Source: CAD feature listing. Evaluate the final solid. Frame: model axes, mm. Coordinates: 2 decimals unless noted, no trailing zeros. Order: outer loops, then holes, each group sorted by start corner. A loop starts at its lowest first (then second) coordinate and runs counter-clockwise, first axis right, second up.
Item 1: Contact query for flat-ended pins moving along their axis: P1, Ø1.5, axis at x = -11, y = 2.5, coming from the -Z side (3 decimals); P2, Ø8, axis at x = -50, z = -52.5, coming from the -Y side; P3, Ø1, axis at y = 1, z = -73, coming from the +X side (3 decimals); P4, Ø1.6, axis at x = 1.5, y = 1, coming from the +Z side (3 decimals). Output: stop coordinate, or through.
Item 2: Section A-A on x = 0. Return the cut outline in (y, z) (3 decimals), then the cut area to 3 significant figures.
Item 3: Mould query, pull axis X, two halves, no side actions, for faces 1 (the flat face through (-68, 0, -46)), 2 (the cylindrical face through (-17.34, 1.61, 78.1)). Classes: released by +X, released by -X, zero draft, split by the parting line, or undercut.
Item 4: Section B-B on z = 0. Return the cut outline in (x, y) (3 decimals), then the cut area to 3 significant figures.
Item 5: Ray query, line 1 (Z direction, x = 0, y = 2.3) (3 decimals); line 2 (Z direction, x = -49.5, y = 3.05). Return the intervals inside material, ascending.
from build123d import *

# Parameters (mm, degrees)
ESQUISSE1_W             = 200
ESQUISSE1_H             = 200
BOSS_EXTRU_1_DEPTH      = 3.175
ESQUISSE2_W             = 3.175
ESQUISSE2_H             = 35
ESQUISSE2_H_2           = 47.5
ENL_V_MAT_EXTRU_1_DEPTH = 3.175
ESQUISSE4_W             = 44.325
ESQUISSE4_H             = 3.175
ESQUISSE4_W_2           = 35
ENL_V_MAT_EXTRU_3_DEPTH = 3.175
ESQUISSE3_R             = 80
ENL_V_MAT_EXTRU_2_DEPTH = 3.175


with BuildPart() as part:
    # Esquisse1 → Boss.-Extru.1 (new body)
    with BuildSketch(Plane(origin=(0, 0, 0), x_dir=(1, 0, 0), z_dir=(0, 1, 0))):
        Rectangle(ESQUISSE1_W, ESQUISSE1_H)
    extrude(amount=BOSS_EXTRU_1_DEPTH)

    # Esquisse2 → Enlèv. mat.-Extru.1 (cut)
    with BuildSketch(Plane(origin=(0, 3.175, 0), x_dir=(1, 0, 0), z_dir=(0, 1, 0))):
        with Locations((-98.4125, 0)):
            Rectangle(ESQUISSE2_W, ESQUISSE2_H)
        with Locations((-98.4125, 76.25)):
            Rectangle(ESQUISSE2_W, ESQUISSE2_H_2)
        with Locations((-98.4125, -76.25)):
            Rectangle(ESQUISSE2_W, ESQUISSE2_H_2)
    enl_v_mat_extru_1 = extrude(amount=-ENL_V_MAT_EXTRU_1_DEPTH, mode=Mode.SUBTRACT)

    # Symétrie1: Enlèv. mat.-Extru.1 across plane
    add(enl_v_mat_extru_1.mirror(Plane(origin=(0, 0, 0), x_dir=(0, 0, 1), z_dir=(1, 0, 0))), mode=Mode.SUBTRACT)

    # Esquisse4 → Enlèv. mat.-Extru.3 (cut)
    with BuildSketch(Plane(origin=(0, 3.175, 0), x_dir=(1, 0, 0), z_dir=(0, 1, 0))):
        with Locations((-74.6625, 98.4125)):
            Rectangle(ESQUISSE4_W, ESQUISSE4_H)
        with Locations((0, 98.4125)):
            Rectangle(ESQUISSE4_W_2, ESQUISSE4_H)
        with Locations((74.6625, 98.4125)):
            Rectangle(ESQUISSE4_W, ESQUISSE4_H)
    enl_v_mat_extru_3 = extrude(amount=-ENL_V_MAT_EXTRU_3_DEPTH, mode=Mode.SUBTRACT)

    # Symétrie2: Enlèv. mat.-Extru.3 across plane
    add(enl_v_mat_extru_3.mirror(Plane.XY), mode=Mode.SUBTRACT)

    # Esquisse3 → Enlèv. mat.-Extru.2 (cut)
    with BuildSketch(Plane(origin=(0, 3.175, 0), x_dir=(1, 0, 0), z_dir=(0, 1, 0))):
        Circle(ESQUISSE3_R)
    extrude(amount=-ENL_V_MAT_EXTRU_2_DEPTH, mode=Mode.SUBTRACT)


solid = part.part
Answer list:
1. P1: stops at z = -96.825
1. P2: passes through
1. P3: stops at x = 96.825
1. P4: stops at z = 96.825
2. outline: (0, -96.825) - (3.175, -96.825) - (3.175, -80) - (0, -80) - close; (0, 80) - (3.175, 80) - (3.175, 96.825) - (0, 96.825) - close
2. area: 107 mm2
3. face 1: zero draft
3. face 2: undercut
4. outline: (-96.825, 0) - (-80, 0) - (-80, 3.175) - (-96.825, 3.175) - close; (80, 0) - (96.825, 0) - (96.825, 3.175) - (80, 3.175) - close
4. area: 107 mm2
5. line 1: z = -96.825 to -80, 80 to 96.825
5. line 2: z = -100 to -62.85, 62.85 to 100
